Part model, mm, in its own coordinate system. A direction names the side the tool comes from. Round coordinates to 2 decimals unless told otherwise and drop trailing zeros. Write each loop counter-clockwise with the first axis right and the second up, starting at its lowest first coordinate (ties: lowest second). Pieces come first, ordered by that corner, then holes.
from build123d import *

# Parameters (mm, degrees)
F1_DEPTH    = 4.572
F2_T1_DEPTH = 4.572
F2_T3_DEPTH = 11.6353556042
F2_T5_DEPTH = 10.2806889376


# Not quite as in the source:
# - a fillet or chamfer that OpenCascade refuses, or shapes differently, is made with other operations: its cross-section is extruded or revolved along the edge and cut away or added


with BuildPart() as f1:
    # F0 (on Top) → F1 (new body)
    with BuildSketch(Plane.XY):
        Polygon((-16.9968333333, -0.15875), (-20.1718333333, -0.15875), (-20.1718333333, -1.42875), (-16.9968333333, -1.42875), (-16.9968333333, -1.5875), (-1.7568333333, -1.5875), (-4.2968333333, -25.4), (-2.7093333333, -25.4), (0, 0), (-16.9968333333, 0), align=None)
    extrude(amount=F1_DEPTH)

    # F2: fillet of radius 1.27 on 4 edges, made by hand

    # F2_s2 → F2_t1 (join)
    with BuildSketch(Plane.XY):
        with BuildLine():
            ThreePointArc((-1.9066682695, -2.9922025264), (-2.2250542944, -2.0084335151), (-3.1695044542, -1.5875))
            Line((-3.1695044542, -1.5875), (-1.7568333333, -1.5875))
            Line((-1.7568333333, -1.5875), (-1.9066682695, -2.9922025264))
        make_face()
    extrude(amount=F2_T1_DEPTH)

    # F2_s4 → F2_t3 (cut)
    with BuildSketch(Plane.XY.offset(-3.5316778021)):
        with BuildLine():
            ThreePointArc((-4.1469983972, -23.9952974736), (-3.8286123722, -24.9790664849), (-2.8841622125, -25.4))
            Line((-2.8841622125, -25.4), (-4.2968333333, -25.4))
            Line((-4.2968333333, -25.4), (-4.1469983972, -23.9952974736))
        make_face()
        with BuildLine():
            ThreePointArc((-0.1498349361, -1.4047025264), (-0.4682209611, -0.4209335151), (-1.4126711208, 0))
            Line((-1.4126711208, 0), (0, 0))
            Line((0, 0), (-0.1498349361, -1.4047025264))
        make_face()
    extrude(amount=F2_T3_DEPTH, mode=Mode.SUBTRACT)

    # F2_s6 → F2_t5 (cut)
    with BuildSketch(Plane.XY.offset(-2.8543444688)):
        with BuildLine():
            ThreePointArc((-3.8510711208, -25.4), (-3.002004636, -25.0744501597), (-2.5882349361, -24.2647025264))
            Line((-2.5882349361, -24.2647025264), (-2.7093333333, -25.4))
            Line((-2.7093333333, -25.4), (-3.8510711208, -25.4))
        make_face()
    extrude(amount=F2_T5_DEPTH, mode=Mode.SUBTRACT)


solid = f1.part
Q1. Wall check: line 1 (Y direction, x = -11.25, z = 2.6); line 2 (Y direction, x = -18.5, z = 4.45); line 3 (X direction, y = -5.75, z = 0.8). Give the ranges that are in metal, low to high.
Q2. Tool access for faces 1 (the flat face through (-19, -0.159, 2)), 2 (the flat face through (-19, -1.429, 2)), 3 (the flat face through (-3.01, -13.35, 2.25)): list every direction of +Z, -Z, +X, -X, +Y, -Y with a clear straight run to the whole face (end or side of a thin tool).
Q3. Drop flat-ended pins along their axis: P1, Ø1.6, axis at x = -18.5, z = 2, coming from the +Y side; P2, Ø1.6, axis at x = -18, z = 1.5, coming from the -Y side; P3, Ø1, axis at y = -18.5, z = 0.5, coming from the -X side. Give the stop position or say it passes through.
Q4. Two-plate mould, pull along Y, no slides. Class faces 4 (the cylindrical face through (-2.215, -2.02, 2.254)), 5 (the flat face through (-2, -7, 4.572)), 6 (the flat face through (-9, 0, 2)): released by +Y, released by -Y, zero draft, split by the parting line, or undercut.
Q5. Saw through at B-B, the plane x = -14. Write the cut outline in (y, z).
Q6. Saw through at C-C, the plane y = -21. Write the cut outline in (x, z).
Q7. Saw through at A-A, the plane z = 4. Write the cut outline in (x, y), and give its area (3 significant figures).
Computed:
1. line 1: y = -1.59 to 0
1. line 2: y = -1.43 to -0.16
1. line 3: x = -2.2 to -0.61
2. face 1: +Z, -Z, -X, +Y
2. face 2: +Z, -Z, -X, -Y
2. face 3: +Z, -Z, -X
3. P1: stops at y = -0.16
3. P2: stops at y = -1.43
3. P3: stops at x = -3.61
4. face 4: undercut
4. face 5: zero draft
4. face 6: released by +Y
5. outline: (-1.59, 0) - (0, 0) - (0, 4.57) - (-1.59, 4.57) - close
6. outline: (-3.83, 0) - (-2.24, 0) - (-2.24, 4.57) - (-3.83, 4.57) - close
7. outline: (-20.17, -1.43) - (-17, -1.43) - (-17, -1.59) - (-3.17, -1.59) arc R1.27 cw to (-1.91, -2.99) - (-4.15, -24) arc R1.27 ccw to (-3.37, -25.3) arc R1.27 ccw to (-2.59, -24.26) - (-0.15, -1.4) arc R1.27 ccw to (-1.41, 0) - (-17, 0) - (-17, -0.16) - (-20.17, -0.16) - close
7. area: 68.0 mm2
